```python
from build123d import *

# Parameters (mm, degrees)
F1_DEPTH = 20
F2_R     = 5
F3_DEPTH = 25
F4_W     = 30
F4_H     = 10.5
F5_DEPTH = 30


with BuildPart() as f1:
    # F0 (on Top) → F1 (new body)
    with BuildSketch(Plane.XY):
        with BuildLine():
            ThreePointArc((40, 0), (35.606602, 10.606602), (25, 15))
            Line((25, 15), (-25, 15))
            ThreePointArc((-25, 15), (-35.606602, 10.606602), (-40, 0))
            ThreePointArc((-40, 0), (-35.606602, -10.606602), (-25, -15))
            Line((-25, -15), (25, -15))
            ThreePointArc((25, -15), (35.606602, -10.606602), (40, 0))
        make_face()
    extrude(amount=F1_DEPTH)

    # F2 (on face) → F3 (cut)
    with BuildSketch(Plane.XY.offset(20)):
        with Locations((25, 0)):
            Circle(F2_R)
        with Locations((-25, 0)):
            Circle(F2_R)
    extrude(amount=-F3_DEPTH, mode=Mode.SUBTRACT)

    # F4 (on face) → F5 (cut)
    with BuildSketch(Plane.XZ.offset(15)):
        with Locations((25, 10)):
            Rectangle(F4_W, F4_H)
        with Locations((-25, 10)):
            Rectangle(F4_W, F4_H)
    extrude(amount=-F5_DEPTH, mode=Mode.SUBTRACT)


solid = f1.part
```
Model file for the job. Use its own axes, mm. A direction names the side the tool comes from. Coordinates: 2 decimals unless noted, no trailing zeros. Write each loop counter-clockwise with the first axis right and the second up, starting at its lowest first coordinate (ties: lowest second). Pieces come first, ordered by that corner, then holes. Notation, with made-up numbers: (-21, 22) - (37, 22) arc R23 cw to (37, 49) - close; hole circle Ø2 at (72, 63.25). An arc over 180 degrees is marked (long way). Use a Markdown table: item, result. Add a question column.
Item 1: Band-saw the part on D-D, the plane z = 8. Write the cut outline in (x, y).
Item 2: Drill centre lines: line 1 along Z through (x, y) = (-12, 7); line 2 along Y through (x, z) = (25, 1.35); line 3 along X through (y, z) = (-1, 3.25). Where is each one in solid material? Low to high.
Item 3: Band-saw the part on A-A, the plane z = 17.5. Write the cut outline in (x, y), and give its area (3 significant figures).
Item 4: Band-saw the part on B-B, the plane y = -1. Write the cut outline in (x, z).
Item 5: 3-axis set-ups, long thin cutter, end or side, ignore diameter. For faces 5 (the face through (-30, 0, 18)), 6 (the face through (-19, 0, 15.25)), 7 (the face through (21, -4, 15.25)): which of +Z, -Z, +X, -X, +Y, -Y reach the whole face in a straight line?
Item 6: Band-saw the part on C-C, the plane y = -12. Write the cut outline in (x, z), and give its area (3 significant figures).
Item 7: Drop flat-ended pins along their axis: pin 1 (11.5 mm diameter, centred on y = 7, z = 7.5, fed in from +X); pin 2 (6 mm diameter, centred on y = 5, z = 4, fed in from -X); pin 3 (5 mm diameter, centred on y = -3.5, z = 8, fed in from -X). Give the stop position or say it passes through.
Item 8: Two-plate mould, pull along Z, no slides. Class faces 1 (the face through (0, -15, 10)), 2 (the face through (-1, 0, 20)), 3 (the face through (10, 0, 10)), 4 (the face through (-10, 0, 10)): pulls with the +Z half, pulls with the -Z half, needs draft (parallel to the pull), parting line crosses it, or undercut.
A:
| question | item | result |
|---|---|---|
| 1 | outline | (-10, -15) - (10, -15) - (10, 15) - (-10, 15) - close |
| 2 | line 1 | z = 0 to 4.75, 15.25 to 20 |
| 2 | line 2 | y = -15 to -5, 5 to 15 |
| 2 | line 3 | x = -39.97 to -29.9, -20.1 to 20.1, 29.9 to 39.97 |
| 3 | outline | (-40, 0) arc R15 ccw to (-25, -15) - (25, -15) arc R15 ccw to (40, 0) arc R15 ccw to (25, 15) - (-25, 15) arc R15 ccw to start; hole circle Ø10 at (-25, 0); hole circle Ø10 at (25, 0) |
| 3 | area | 2,050 mm² |
| 4 | outline | (-39.97, 0) - (-29.9, 0) - (-29.9, 4.75) - (-39.97, 4.75) - close; (-39.97, 15.25) - (-29.9, 15.25) - (-29.9, 20) - (-39.97, 20) - close; (-20.1, 0) - (20.1, 0) - (20.1, 4.75) - (10, 4.75) - (10, 15.25) - (20.1, 15.25) - (20.1, 20) - (-20.1, 20) - (-20.1, 15.25) - (-10, 15.25) - (-10, 4.75) - (-20.1, 4.75) - close; (29.9, 0) - (39.97, 0) - (39.97, 4.75) - (29.9, 4.75) - close; (29.9, 15.25) - (39.97, 15.25) - (39.97, 20) - (29.9, 20) - close |
| 5 | face 5 | +Z, -Z |
| 5 | face 6 | -X, +Y, -Y |
| 5 | face 7 | +X, +Y, -Y |
| 6 | outline | (-34, 0) - (34, 0) - (34, 4.75) - (10, 4.75) - (10, 15.25) - (34, 15.25) - (34, 20) - (-34, 20) - (-34, 15.25) - (-10, 15.25) - (-10, 4.75) - (-34, 4.75) - close |
| 6 | area | 856 mm² |
| 7 | pin 1 | stops at x = 39.87 |
| 7 | pin 2 | stops at x = -39.87 |
| 7 | pin 3 | stops at x = -10 |
| 8 | face 1 | needs draft |
| 8 | face 2 | pulls with the +Z half |
| 8 | face 3 | undercut |
| 8 | face 4 | undercut |
